Geometry: final body of the model. Coordinates: model frame, mm. Give positions to 0.01 mm unless a question says otherwise; leave off trailing zeros. Answer as a JSON object with one key per item and string values.
Autodesk Inventor part; units mm, degrees
ref_plane "side_4d_XY" through (-20, 0, -286) normal (-1, 0, 0) x (0, 1, 0)
ref_plane "side_4d_YZ" through (-20, 0, -286) normal (0, 1, 0) x (0, 0, -1)
ref_plane "side_4d_ZX" through (-20, 0, -286) normal (0, 0, -1) x (-1, 0, 0)
sketch "Skizze_1" plane through (0, 0, 0) normal (0, 0, 1) x (1, 0, 0)
  arc A0 (-20, -17) -> (-17, -20) centre (-17, -17) ccw
  line L0 (-17, -20) -> (-4.1, -20)
  line L1 (-4.1, -20) -> (-4.1, -17)
  line L2 (-4.1, -17) -> (-10.5, -17)
  line L3 (-10.5, -17) -> (-10.5, -13.6627)
  arc A1 (-10.0314, -12.5314) -> (-10.5, -13.6627) centre (-8.9002, -13.6627) ccw
  line L4 (-10.0314, -12.5314) -> (-7.4645, -9.9645)
  arc A2 (-3.9289, -8.5) -> (-7.4645, -9.9645) centre (-3.9289, -13.5) ccw
  line L5 (-3.9289, -8.5) -> (3.9289, -8.5)
  arc A3 (7.4645, -9.9645) -> (3.9289, -8.5) centre (3.9289, -13.5) ccw
  line L6 (7.4645, -9.9645) -> (10.0314, -12.5314)
  arc A4 (10.5, -13.6627) -> (10.0314, -12.5314) centre (8.9002, -13.6627) ccw
  line L7 (10.5, -13.6627) -> (10.5, -17)
  line L8 (10.5, -17) -> (4.1, -17)
  line L9 (4.1, -17) -> (4.1, -20)
  line L10 (4.1, -20) -> (17, -20)
  arc A5 (17, -20) -> (20, -17) centre (17, -17) ccw
  line L11 (20, -17) -> (20, -4.1)
  line L12 (20, -4.1) -> (17, -4.1)
  line L13 (17, -4.1) -> (17, -10.5)
  line L14 (17, -10.5) -> (13.6627, -10.5)
  arc A6 (12.5314, -10.0314) -> (13.6627, -10.5) centre (13.6627, -8.9002) ccw
  line L15 (12.5314, -10.0314) -> (9.9645, -7.4645)
  arc A7 (8.5, -3.9289) -> (9.9645, -7.4645) centre (13.5, -3.9289) ccw
  line L16 (8.5, -3.9289) -> (8.5, 3.9289)
  arc A8 (9.9645, 7.4645) -> (8.5, 3.9289) centre (13.5, 3.9289) ccw
  line L17 (9.9645, 7.4645) -> (12.5314, 10.0314)
  arc A9 (13.6627, 10.5) -> (12.5314, 10.0314) centre (13.6627, 8.9002) ccw
  line L18 (13.6627, 10.5) -> (17, 10.5)
  line L19 (17, 10.5) -> (17, 4.1)
  line L20 (17, 4.1) -> (20, 4.1)
  line L21 (20, 4.1) -> (20, 17)
  arc A10 (20, 17) -> (17, 20) centre (17, 17) ccw
  line L22 (17, 20) -> (4.1, 20)
  line L23 (4.1, 20) -> (4.1, 17)
  line L24 (4.1, 17) -> (10.5, 17)
  line L25 (10.5, 17) -> (10.5, 13.6627)
  arc A11 (10.0314, 12.5314) -> (10.5, 13.6627) centre (8.9002, 13.6627) ccw
  line L26 (10.0314, 12.5314) -> (7.4645, 9.9645)
  arc A12 (3.9289, 8.5) -> (7.4645, 9.9645) centre (3.9289, 13.5) ccw
  line L27 (3.9289, 8.5) -> (-3.9289, 8.5)
  arc A13 (-7.4645, 9.9645) -> (-3.9289, 8.5) centre (-3.9289, 13.5) ccw
  line L28 (-7.4645, 9.9645) -> (-10.0314, 12.5314)
  arc A14 (-10.5, 13.6627) -> (-10.0314, 12.5314) centre (-8.9002, 13.6627) ccw
  line L29 (-10.5, 13.6627) -> (-10.5, 17)
  line L30 (-10.5, 17) -> (-4.1, 17)
  line L31 (-4.1, 17) -> (-4.1, 20)
  line L32 (-4.1, 20) -> (-17, 20)
  arc A15 (-17, 20) -> (-20, 17) centre (-17, 17) ccw
  line L33 (-20, 17) -> (-20, 4.1)
  line L34 (-20, 4.1) -> (-17, 4.1)
  line L35 (-17, 4.1) -> (-17, 10.5)
  line L36 (-17, 10.5) -> (-13.6627, 10.5)
  arc A16 (-12.5314, 10.0314) -> (-13.6627, 10.5) centre (-13.6627, 8.9002) ccw
  line L37 (-12.5314, 10.0314) -> (-9.9645, 7.4645)
  arc A17 (-8.5, 3.9289) -> (-9.9645, 7.4645) centre (-13.5, 3.9289) ccw
  line L38 (-8.5, 3.9289) -> (-8.5, -3.9289)
  arc A18 (-9.9645, -7.4645) -> (-8.5, -3.9289) centre (-13.5, -3.9289) ccw
  line L39 (-9.9645, -7.4645) -> (-12.5314, -10.0314)
  arc A19 (-13.6627, -10.5) -> (-12.5314, -10.0314) centre (-13.6627, -8.9002) ccw
  line L40 (-13.6627, -10.5) -> (-17, -10.5)
  line L41 (-17, -10.5) -> (-17, -4.1)
  line L42 (-17, -4.1) -> (-20, -4.1)
  line L43 (-20, -4.1) -> (-20, -17)
  circle A20 centre (0, 0) radius 6
extrude "Extrusion1" add sketch "Skizze_1" against normal blind 572
sketch "Sketch2" plane through (0, 0, 0) normal (0, 0, 1) x (1, 0, 0)
  point P0 (-15, -15)
hole "Drilling 1" at (-15, -15, 0) direction (0, 0, -1) diameter 5 depth 6000
sketch "Sketch3" plane through (0, 0, 0) normal (0, 0, 1) x (1, 0, 0)
  point P0 (15, -15)
hole "Drilling 2" at (15, -15, 0) direction (0, 0, -1) diameter 5 depth 6000
sketch "Sketch4" plane through (0, 0, 0) normal (0, 0, 1) x (1, 0, 0)
  point P0 (15, 15)
hole "Drilling 3" at (15, 15, 0) direction (0, 0, -1) diameter 5 depth 6000
sketch "Sketch5" plane through (0, 0, 0) normal (0, 0, 1) x (1, 0, 0)
  point P0 (-15, 15)
hole "Drilling 4" at (-15, 15, 0) direction (0, 0, -1) diameter 5 depth 6000
ref_plane "side_4d_XY" through (-20, 0, -286) normal (-1, 0, 0) x (0, 1, 0)
ref_plane "side_4d_YZ" through (-20, 0, -286) normal (0, 1, 0) x (0, 0, -1)
ref_plane "side_4d_ZX" through (-20, 0, -286) normal (0, 0, -1) x (-1, 0, 0)
ref_plane "side_1a_XY" through (0, 20, -286) normal (0, 1, 0) x (1, 0, 0)
ref_plane "side_1a_YZ" through (0, 20, -286) normal (1, 0, 0) x (0, 0, -1)
ref_plane "side_1a_ZX" through (0, 20, -286) normal (0, 0, -1) x (0, 1, 0)
ref_plane "side_2b_XY" through (20, 0, -286) normal (1, 0, 0) x (0, -1, 0)
ref_plane "side_2b_YZ" through (20, 0, -286) normal (0, -1, 0) x (0, 0, -1)
ref_plane "side_2b_ZX" through (20, 0, -286) normal (0, 0, -1) x (1, 0, 0)
ref_plane "side_3c_XY" through (0, -20, -286) normal (0, -1, 0) x (-1, 0, 0)
ref_plane "side_3c_YZ" through (0, -20, -286) normal (-1, 0, 0) x (0, 0, -1)
ref_plane "side_3c_ZX" through (0, -20, -286) normal (0, 0, -1) x (0, -1, 0)
ref_plane "end_XY" through (0, 0, -572) normal (0, 0, -1) x (1, 0, 0)
ref_plane "end_YZ" through (0, 0, -572) normal (1, 0, 0) x (0, -1, 0)
ref_plane "end_ZX" through (0, 0, -572) normal (0, -1, 0) x (0, 0, -1)
ref_plane "start_XY" through (0, 0, 0) normal (0, 0, 1) x (1, 0, 0)
ref_plane "start_YZ" through (0, 0, 0) normal (1, 0, 0) x (0, 1, 0)
ref_plane "start_ZX" through (0, 0, 0) normal (0, 1, 0) x (0, 0, 1)
properties part number "MayTec 1.11.040040.43S_Profile 40x40, 4E, S_572_Detail_(0;0,0,0)"
1) Contact query for flat-ended pins moving along their axis: P1, Ø3, axis at x = 15, y = -15, coming from the +Z side; P2, Ø0.9, axis at x = -18.5, z = -250, coming from the -Y side; P3, Ø5, axis at y = 0.5, z = -207.5, coming from the +X side; P4, Ø2, axis at y = 0.5, z = -154, coming from the -X side. Output: stop coordinate, or through.
Geometry check:
{"P1": "passes through", "P2": "stops at y = -19.81", "P3": "stops at x = 8.5", "P4": "stops at x = -8.5"}
2) Line query: line 1 (X direction, y = -4.5, z = -153.5); line 2 (X direction, y = 15, z = -310); line 3 (X direction, y = -8, z = -192.5). Output: solid intervals per line, ascending. Write a range as from..to.
Geometry check:
{"line 1": "x = -20..-17, -8.53..-3.97, 3.97..8.53, 17..20", "line 2": "x = -20..-17.5, -12.5..-10.5, 10.5..12.5, 17.5..20", "line 3": "x = -20..-17, -10.5..10.5, 17..20"}
3) Cut plane A-A on z = -492. Give the number of separate pieces and of enclosed holes in the cut face, and give its area (3 significant figures).
Geometry check:
{"separate pieces": "1", "enclosed holes": "5", "area": "674 mm2"}
4) Pull-direction query (Y, two-part tool) for faces 1 (the cylindrical face through (-6, 0, -282)), 2 (the flat face through (-5, -4, -572)), 3 (the flat face through (11, 20, -282)); classes: pulls with the +Y half, pulls with the -Y half, needs draft (parallel to the pull), parting line crosses it, or undercut.
Geometry check:
{"face 1": "undercut", "face 2": "needs draft", "face 3": "pulls with the +Y half"}
